Autodesk Inventor part; units mm, degrees
ref_plane "YZ Plane" through (0, 0, 0) normal (1, 0, 0) x (0, 1, 0)
ref_plane "XZ Plane" through (0, 0, 0) normal (0, 1, 0) x (-1, 0, 0)
ref_plane "XY Plane" through (0, 0, 0) normal (0, 0, 1) x (1, 0, 0)
sketch "Sketch1" plane through (0, 0, 0) normal (0, 1, 0) x (-1, 0, 0)
  circle A0 centre (0, 0) radius 3.95
  circle A1 centre (0, 0) radius 7
  dimension "d0" = 7.9
  dimension "d1" = 14
extrude "Extrusion1" add sketch "Sketch1" along normal blind 250 contours A0
sketch "Sketch2" plane through (0, 250, 0) normal (0, 1, 0) x (1, 0, 0)
  circle A0 centre (0, 0) radius 3.95
  circle A1 centre (0, 0) radius 7
  dimension "d4" = 14
extrude "Extrusion2" add sketch "Sketch2" against normal blind 7
sketch "Sketch3" plane through (0, 0, 0) normal (0, -1, 0) x (1, 0, 0)
  circle A0 centre (0, 0) radius 7
  circle A1 centre (0, 0) radius 7
extrude "Extrusion3" add sketch "Sketch3" against normal blind 7
thread "Thread1"
properties part number "perno"
Here's how the part is built. I have some questions about the finished solid (model axes, mm). A direction names the side the tool comes from. Give positions to 0.01 mm unless a question says otherwise; leave off trailing zeros. Loops run counter-clockwise (first coordinate to the right, second up) from the corner with the lowest first, then second, coordinate; pieces in that order, holes last. Notation, with made-up numbers: (44, 52) -> (100, 52) arc R11 ccw to (100, 67) -> close; hole circle Ø10 at (78, 82). An arc over 180 degrees is marked (long way). Answer as a JSON object with one key per item and string values. Group by question number.
Item 1: On a 3-axis mill with a long thin cutter (end or side, diameter ignored), from which of +Z, -Z, +X, -X, +Y, -Y can I reach the whole of each face in a straight line? I mean faces 5 (the flat face through (0, 0, 0)), 6 (the cylindrical face through (3.135, 123.348, 2.404)). Say none if no direction works.
Item 2: Imagine slicing it at A-A on x = 0. Write out the boundary of the cut face in (y, z).
Item 3: Will these pins go through, and if not, where does the flat tip stop? pin 1 (5 mm diameter, centred on y = 29, z = 5.5, fed in from +X); pin 2 (8 mm diameter, centred on y = 80, z = 0.5, fed in from +X); pin 3 (2 mm diameter, centred on y = 38, z = 1, fed in from -X); pin 4 (2 mm diameter, centred on y = 58.5, z = -5, fed in from +X).
Item 4: Imagine slicing it at C-C on y = 58.5. Write out the boundary of the cut face in (x, z).
Item 5: Imagine slicing it at B-B on z = 0. Write out the boundary of the cut face in (x, y).
Item 6: Thinking about a two-plate mould opening in Y: for faces 1 (the cylindrical face through (6.466, 246.549, 2.681)), 2 (the flat face through (3, 243, 3)), 3 (the flat face through (3, 7, -3)), 4 (the flat face through (0, 250, 0)), which applies, pulls with the +Y half, pulls with the -Y half, needs draft (parallel to the pull), parting line crosses it, or undercut?
Item 7: I need wall thicknesses on L1, parallel to Y at x = 1.25, z = -5.75; L2, parallel to X at y = 185, z = 0.25. Which ranges of each line are inside material? Lowest first, please.
Answer list:
{
 "1": {"face 5": "+Z, -Z, +X, -X, -Y", "face 6": "none"},
 "2": {"outline": "(0, -7) -> (7, -7) -> (7, -3.95) -> (243, -3.95) -> (243, -7) -> (250, -7) -> (250, 7) -> (243, 7) -> (243, 3.95) -> (7, 3.95) -> (7, 7) -> (0, 7) -> close"},
 "3": {"pin 1": "stops at x = 2.57", "pin 2": "stops at x = 3.95", "pin 3": "stops at x = -3.95", "pin 4": "passes through"},
 "4": {"outline": "circle Ø7.9 at (0, 0)"},
 "5": {"outline": "(-7, 0) -> (7, 0) -> (7, 7) -> (3.95, 7) -> (3.95, 243) -> (7, 243) -> (7, 250) -> (-7, 250) -> (-7, 243) -> (-3.95, 243) -> (-3.95, 7) -> (-7, 7) -> close"},
 "6": {"face 1": "needs draft", "face 2": "undercut", "face 3": "undercut", "face 4": "pulls with the +Y half"},
 "7": {"L1": "y = 0 to 7, 243 to 250", "L2": "x = -3.94 to 3.94"}
}
